The figure shows three views and two pictorial views of one solid part (mm, origin at its lowest corner). Answer the questions. Give positions to 0.01 mm unless a question says otherwise; leave off trailing zeros. Loops run counter-clockwise (first coordinate to the right, second up) from the corner with the lowest first, then second, coordinate; pieces in that order, holes last. Notation, with made-up numbers: (-19.75, -32) - (39.25, -32) arc R7 cw to (39.25, -23) - close; hole circle Ø7 at (18.25, 28.25). An arc over 180 degrees is marked (long way). Write item = value, one per line.
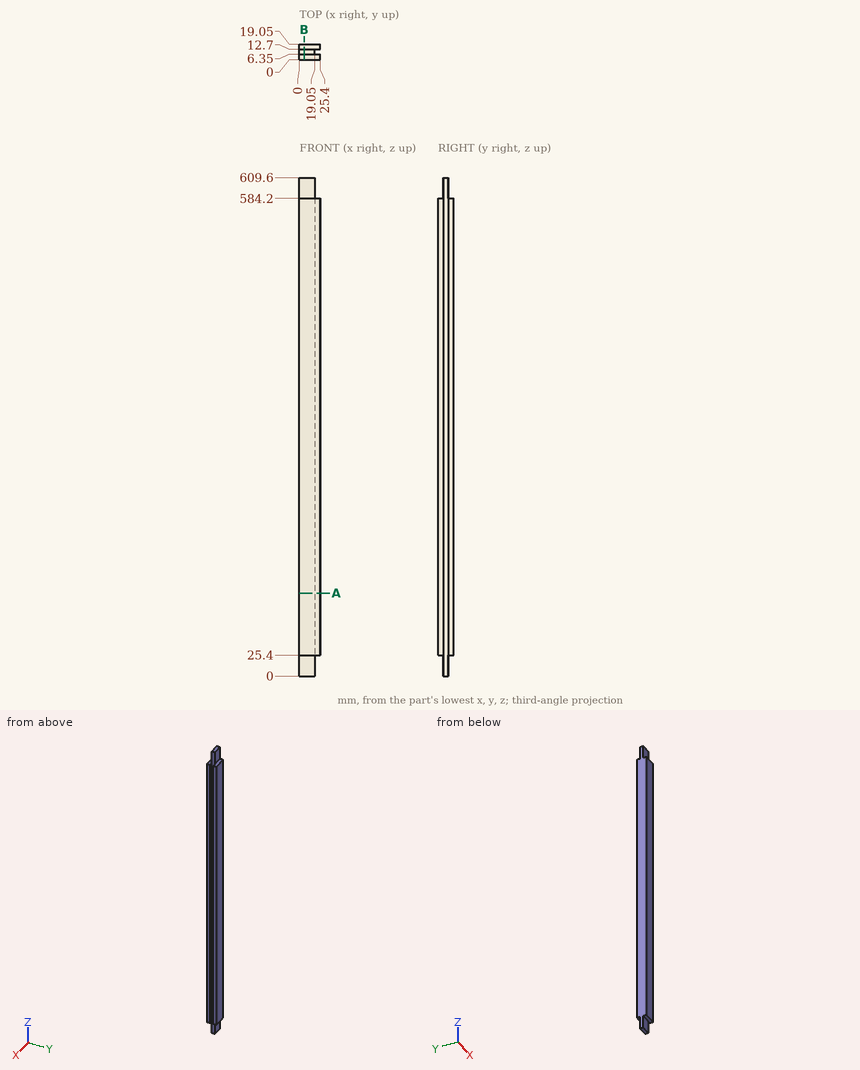
1) A cutting plane is placed at A-A on z = 101.5. Determine the outline of the cut face in (x, y), then the cut area to 3 significant figures.
Output:
outline = (0, 0) - (25.4, 0) - (25.4, 6.35) - (19.05, 6.35) - (19.05, 12.7) - (25.4, 12.7) - (25.4, 19.05) - (0, 19.05) - close
area = 444 mm²
2) Each of these flat-tipped pins is pushed along its axis until it touches: P1, Ø5, axis at x = 16, y = 17, coming from the +Z side; P2, Ø5.5, axis at x = 12, z = 595, coming from the +Y side; P3, Ø3, axis at x = 7, y = 17, coming from the -Z side. Where does it stop, or does it pass through?
Output:
P1 = 584.2
P2 = 12.7
P3 = 25.4
3) A cutting plane is placed at B-B on x = 5.75. Determine the outline of the cut face in (y, z), then the cut area to 3 significant figures.
Output:
outline = (0, 25.4) - (6.35, 25.4) - (6.35, 0) - (12.7, 0) - (12.7, 25.4) - (19.05, 25.4) - (19.05, 584.2) - (12.7, 584.2) - (12.7, 609.6) - (6.35, 609.6) - (6.35, 584.2) - (0, 584.2) - close
area = 11,000 mm²
4) Find the intervals of material crossed by probe 1 along Y at (x, z) = (23, 36.5); probe 2 along Z at (x, y) = (11.5, 14.5); probe 3 along X at (y, z) = (7, 285), in increasing order.
Output:
probe_1 = 0 to 6.35, 12.7 to 19.05
probe_2 = 25.4 to 584.2
probe_3 = 0 to 19.05
